Geometry: final body of the model. Coordinates: model frame, mm. Coordinates: 2 decimals unless noted, no trailing zeros. Order: outer loops, then holes, each group sorted by start corner. A loop starts at its lowest first (then second) coordinate and runs counter-clockwise, first axis right, second up. Notation, with made-up numbers: M 2,20.5 L 10,20.5 A29 ccw 10,43.5 Z; hole C 39.5,11 d7. An arc over 180 degrees is marked long. Use CSV: the item, a comma, the result in double quotes. Start each with the question number.
Q1. Section query D-D, the plane y = -5.25. Output: boundary loops of the cut face in (x, z), and give its area (3 significant figures).
Q2. Section query C-C, the plane x = -13. Output: boundary loops of the cut face in (y, z), and give its area (3 significant figures).
Q3. Section query B-B, the plane z = 20. Output: boundary loops of the cut face in (x, y).
Q4. Ray query, probe 1 along Z at (x, y) = (-1, -11.3); probe 2 along Z at (x, y) = (-13.25, -12.25); probe 3 along Y at (x, z) = (0, -12). Return the intervals inside material, ascending.
Q5. First-contact query: P1, Ø5, axis at y = 11.3, z = 20, coming from the -X side. Flat tip, straight axial feed; report the tip coordinate or a pass-through.
Q6. Section query A-A, the plane x = 0. Output: boundary loops of the cut face in (y, z), and give its area (3 significant figures).
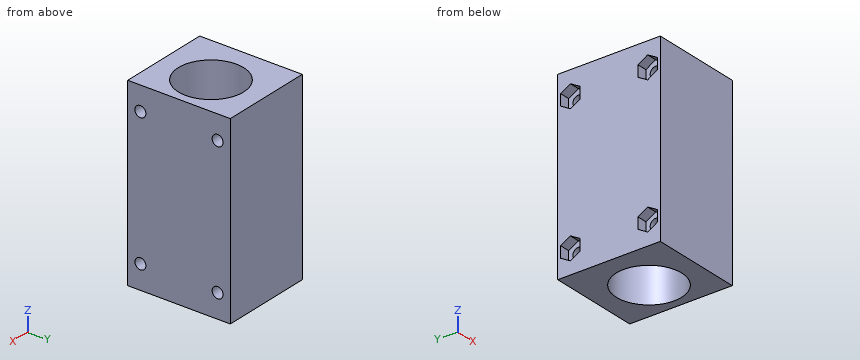
from build123d import *

# Parameters (mm, degrees)
F0_W     = 27
F0_H     = 30
F0_R     = 9.55
F1_DEPTH = 27
F2_R     = 1.6
F3_DEPTH = 27.001
F5_DEPTH = 3


with BuildPart() as f1:
    # F0 (on Top) → F1 (new body, symmetric)
    with BuildSketch(Plane.XY):
        with Locations((-1.5, 0)):
            Rectangle(F0_W, F0_H)
        Circle(F0_R, mode=Mode.SUBTRACT)
    extrude(amount=F1_DEPTH, both=True)

    # F2 (on face) → F3 (cut, through all)
    with BuildSketch(Plane.YZ.offset(12)):
        with Locations((11.3, 20)):
            Circle(F2_R)
        with Locations((11.3, -20)):
            Circle(F2_R)
        with Locations((-11.3, 20)):
            Circle(F2_R)
        with Locations((-11.3, -20)):
            Circle(F2_R)
    extrude(amount=-F3_DEPTH, mode=Mode.SUBTRACT)

    # F4 (on face) → F5 (cut)
    with BuildSketch(Plane(origin=(-15, 0, 0), x_dir=(0, -1, 0), z_dir=(-1, 0, 0))):
        Polygon((-11.3, -16.7091034656), (-14.15, -18.3545517328), (-14.15, -21.6454482672), (-11.3, -23.2908965344), (-8.45, -21.6454482672), (-8.45, -18.3545517328), align=None)
        Polygon((-11.3, 16.7091034656), (-8.45, 18.3545517328), (-8.45, 21.6454482672), (-11.3, 23.2908965344), (-14.15, 21.6454482672), (-14.15, 18.3545517328), align=None)
        Polygon((11.3, -16.7091034656), (8.45, -18.3545517328), (8.45, -21.6454482672), (11.3, -23.2908965344), (14.15, -21.6454482672), (14.15, -18.3545517328), align=None)
        Polygon((8.45, 18.3545517328), (11.3, 16.7091034656), (14.15, 18.3545517328), (14.15, 21.6454482672), (11.3, 23.2908965344), (8.45, 21.6454482672), align=None)
    extrude(amount=-F5_DEPTH, mode=Mode.SUBTRACT)


solid = f1.part
Responses:
1,outline,"M -15,-27 L -7.98,-27 L -7.98,27 L -15,27 Z; M 7.98,-27 L 12,-27 L 12,27 L 7.98,27 Z"
1,area,"596 mm²"
2,outline,"M -15,-27 L 15,-27 L 15,27 L -15,27 Z; hole M -14.15,-21.65 L -11.3,-23.29 L -8.45,-21.65 L -8.45,-18.35 L -11.3,-16.71 L -14.15,-18.35 Z; hole M -14.15,18.35 L -11.3,16.71 L -8.45,18.35 L -8.45,21.65 L -11.3,23.29 L -14.15,21.65 Z; hole M 8.45,-21.65 L 11.3,-23.29 L 14.15,-21.65 L 14.15,-18.35 L 11.3,-16.71 L 8.45,-18.35 Z; hole M 8.45,18.35 L 11.3,16.71 L 14.15,18.35 L 14.15,21.65 L 11.3,23.29 L 8.45,21.65 Z"
2,area,"1,510 mm²"
3,outline,"M -15,-15 L 12,-15 L 12,-12.9 L -12,-12.9 L -12,-14.15 L -15,-14.15 Z; M -15,-8.45 L -12,-8.45 L -12,-9.7 L 12,-9.7 L 12,9.7 L -12,9.7 L -12,8.45 L -15,8.45 Z; M -15,14.15 L -12,14.15 L -12,12.9 L 12,12.9 L 12,15 L -15,15 Z; hole C 0,0 d19.1"
4,probe 1,"z = -27 to -21.6, -18.4 to 18.4, 21.6 to 27"
4,probe 2,"z = -27 to -22.74, -17.26 to 17.26, 22.74 to 27"
4,probe 3,"y = -15 to -9.55, 9.55 to 15"
5,P1,"stops at x = -12"
6,outline,"M -15,-27 L -9.55,-27 L -9.55,27 L -15,27 Z; M 9.55,-27 L 15,-27 L 15,27 L 9.55,27 Z; hole C -11.3,-20 d3.2; hole C -11.3,20 d3.2; hole C 11.3,-20 d3.2; hole C 11.3,20 d3.2"
6,area,"556 mm²"
